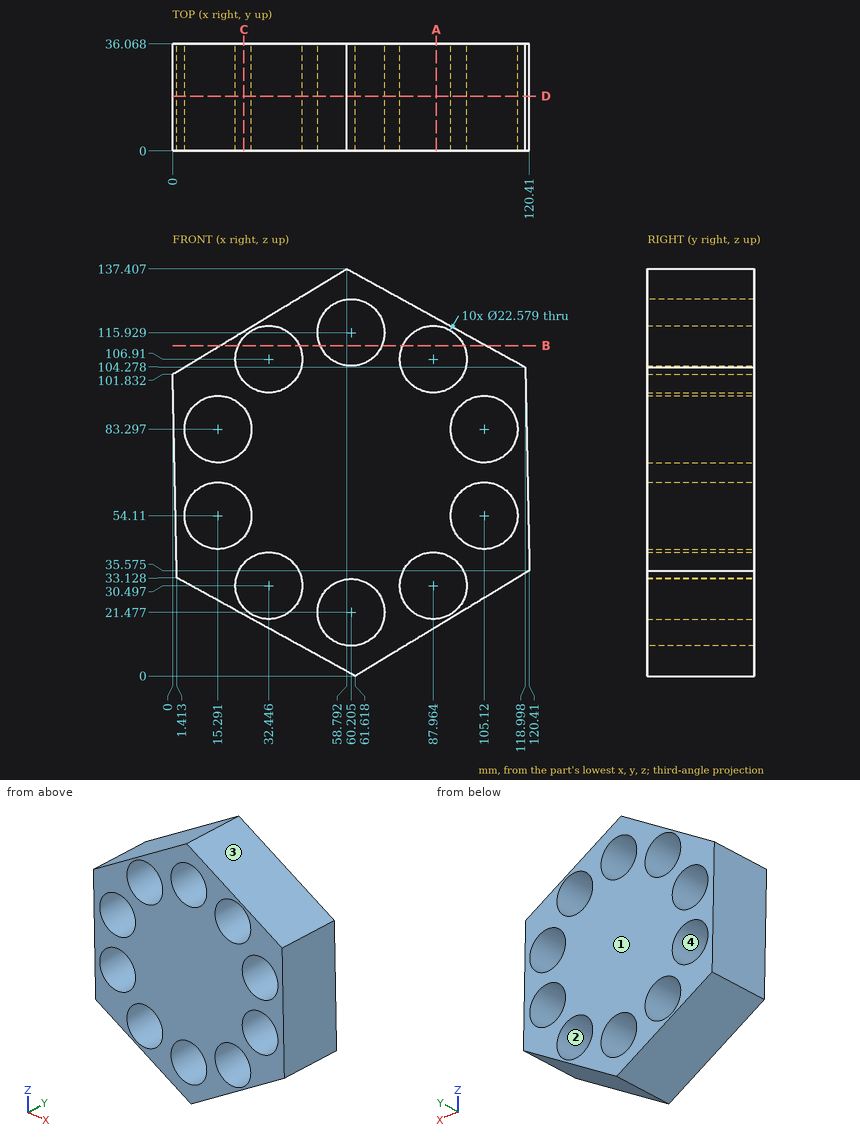
Drawing for the job (mm, zero at the part's lowest x, y, z). Round coordinates to 2 decimals unless told otherwise and drop trailing zeros. Loops run counter-clockwise (first coordinate to the right, second up) from the corner with the lowest first, then second, coordinate; pieces in that order, holes last. Notation, with made-up numbers: M 41.25,-31 L 89.25,-31 A16 ccw 89.25,-8 Z; hole C -17,73.25 d11. An arc over 180 degrees is marked long. Use a Markdown table: item, result. Add a question column.
(1) Pull direction Z, two halves, no side cores. Call the marked faces 1, 2, 3 and 4: +Z half, -Z half, draft (parallel to the pull), parting line (faces both ways), or undercut.
(2) Drill centre lines: line 1 (X direction, y = 26, z = 58.5); line 2 (Z direction, x = 35.5, y = 18) (1 decimal); line 3 (Z direction, x = 88.5, y = 3.5) (1 decimal). Where is each one in solid material? Low to high.
(3) Cut at A-A (x = 89). Give the cut face in (y, z) (1 decimal).
(4) Cut at C-C (x = 24). Give the cut face in (y, z), and give its area (3 significant figures).
(5) Flat gauge pins, fed straight in: pin 1 (6 mm diameter, centred on y = 15.5, z = 21.5, fed in from -X) (1 decimal); pin 2 (12 mm diameter, centred on y = 6, z = 33.5, fed in from +X); pin 3 (8 mm diameter, centred on x = 28.5, y = 7, fed in from +Z). Where does each tip first touch, or does it go through?
(6) Cut at D-D (y = 18.5). State how many separate pieces and enclosed holes the cut face has.
(7) Cut at B-B (z = 111.5). Give the cut face in (x, y).
Geometry says:
| question | item | result |
|---|---|---|
| 1 | face 1 | draft |
| 1 | face 2 | undercut |
| 1 | face 3 | +Z half |
| 1 | face 4 | undercut |
| 2 | line 1 | x = 0.89 to 4.89, 25.69 to 94.72, 115.52 to 119.94 |
| 2 | line 2 | z = 14.4 to 19.6, 41.4 to 96, 117.8 to 123.3 |
| 2 | line 3 | z = 16.3 to 19.2, 41.8 to 95.6, 118.2 to 121.1 |
| 3 | outline | M 0,16.6 L 36.1,16.6 L 36.1,19.3 L 0,19.3 Z; M 0,41.7 L 36.1,41.7 L 36.1,95.7 L 0,95.7 Z; M 0,118.2 L 36.1,118.2 L 36.1,120.8 L 0,120.8 Z |
| 4 | outline | M 0,20.7 L 36.07,20.7 L 36.07,23.01 L 0,23.01 Z; M 0,37.99 L 36.07,37.99 L 36.07,46.93 L 0,46.93 Z; M 0,61.29 L 36.07,61.29 L 36.07,76.11 L 0,76.11 Z; M 0,90.48 L 36.07,90.48 L 36.07,99.42 L 0,99.42 Z; M 0,114.4 L 36.07,114.4 L 36.07,116.35 L 0,116.35 Z |
| 4 | area | 1,330 mm² |
| 5 | pin 1 | stops at x = 17.1 |
| 5 | pin 2 | stops at x = 120.41 |
| 5 | pin 3 | stops at z = 121.5 |
| 6 | separate pieces | 1 |
| 6 | enclosed holes | 10 |
| 7 | outline | M 15.98,0 L 22.13,0 L 22.13,36.07 L 15.98,36.07 Z; M 42.76,0 L 49.82,0 L 49.82,36.07 L 42.76,36.07 Z; M 70.59,0 L 77.65,0 L 77.65,36.07 L 70.59,36.07 Z; M 98.28,0 L 105.87,0 L 105.87,36.07 L 98.28,36.07 Z |
